```python
from build123d import *

# Parameters (mm, degrees)
MODEL_R             = 42.5
MODEL_R_2           = 5.5
MODEL_R_3           = 2.75
MODEL_R_4           = 3.1
MODEL_W             = 25.4
MODEL_H             = 25.4
BOSS_EXTRUDE1_DEPTH = 6.6


with BuildPart() as part:
    # Model → Boss-Extrude1 (new body)
    with BuildSketch(Plane.XY):
        with BuildLine():
            Line((187.8, 2), (187.8, 24.665))
            Line((187.8, 24.665), (176.8, 24.665))
            Line((176.8, 24.665), (176.8, 23.08))
            ThreePointArc((176.8, 23.08), (176.653553391, 22.726446609), (176.3, 22.58))
            Line((176.3, 22.58), (172.3, 22.58))
            ThreePointArc((172.3, 22.58), (171.946446609, 22.726446609), (171.8, 23.08))
            Line((171.8, 23.08), (171.8, 24.665))
            Line((171.8, 24.665), (167.3, 24.665))
            ThreePointArc((167.3, 24.665), (166.946446609, 24.811446609), (166.8, 25.165))
            Line((166.8, 25.165), (166.8, 27.715))
            ThreePointArc((166.8, 27.715), (166.946446609, 28.068553391), (167.3, 28.215))
            Line((167.3, 28.215), (171.8, 28.215))
            Line((171.8, 28.215), (171.8, 29.8))
            ThreePointArc((171.8, 29.8), (171.946446609, 30.153553391), (172.3, 30.3))
            Line((172.3, 30.3), (176.3, 30.3))
            ThreePointArc((176.3, 30.3), (176.653553391, 30.153553391), (176.8, 29.8))
            Line((176.8, 29.8), (176.8, 28.215))
            Line((176.8, 28.215), (187.8, 28.215))
            Line((187.8, 28.215), (187.8, 42.8))
            Line((187.8, 42.8), (191.8, 42.8))
            ThreePointArc((191.8, 42.8), (193.567766953, 43.532233047), (194.3, 45.3))
            Line((194.3, 45.3), (194.3, 55.3))
            ThreePointArc((194.3, 55.3), (193.567766953, 57.067766953), (191.8, 57.8))
            Line((191.8, 57.8), (187.8, 57.8))
            Line((187.8, 57.8), (187.8, 118.92))
            Line((187.8, 118.92), (191.8, 118.92))
            ThreePointArc((191.8, 118.92), (193.567766953, 119.652233047), (194.3, 121.42))
            Line((194.3, 121.42), (194.3, 131.42))
            ThreePointArc((194.3, 131.42), (193.567766953, 133.187766953), (191.8, 133.92))
            Line((191.8, 133.92), (187.8, 133.92))
            Line((187.8, 133.92), (187.8, 152.92))
            Line((187.8, 152.92), (176.8, 152.92))
            Line((176.8, 152.92), (176.8, 151.335))
            ThreePointArc((176.8, 151.335), (176.653553391, 150.981446609), (176.3, 150.835))
            Line((176.3, 150.835), (172.3, 150.835))
            ThreePointArc((172.3, 150.835), (171.946446609, 150.981446609), (171.8, 151.335))
            Line((171.8, 151.335), (171.8, 152.92))
            Line((171.8, 152.92), (167.3, 152.92))
            ThreePointArc((167.3, 152.92), (166.946446609, 153.066446609), (166.8, 153.42))
            Line((166.8, 153.42), (166.8, 155.97))
            ThreePointArc((166.8, 155.97), (166.946446609, 156.323553391), (167.3, 156.47))
            Line((167.3, 156.47), (171.8, 156.47))
            Line((171.8, 156.47), (171.8, 158.055))
            ThreePointArc((171.8, 158.055), (171.946446609, 158.408553391), (172.3, 158.555))
            Line((172.3, 158.555), (176.3, 158.555))
            ThreePointArc((176.3, 158.555), (176.653553391, 158.408553391), (176.8, 158.055))
            Line((176.8, 158.055), (176.8, 156.47))
            Line((176.8, 156.47), (187.8, 156.47))
            Line((187.8, 156.47), (187.8, 169.42))
            Line((187.8, 169.42), (185.8, 171.42))
            Line((185.8, 171.42), (113.770001664, 171.42))
            Line((113.770001664, 171.42), (113.770001664, 158.72))
            Line((113.770001664, 158.72), (106.910001664, 158.72))
            Line((106.910001664, 158.72), (106.910001664, 171.42))
            Line((106.910001664, 171.42), (81.510001665, 171.42))
            Line((81.510001665, 171.42), (81.510001665, 158.72))
            Line((81.510001665, 158.72), (74.650001665, 158.72))
            Line((74.650001665, 158.72), (74.650001665, 171.42))
            Line((74.650001665, 171.42), (2, 171.42))
            Line((2, 171.42), (0, 169.42))
            Line((0, 169.42), (0, 156.47))
            Line((0, 156.47), (11, 156.47))
            Line((11, 156.47), (11, 158.055))
            ThreePointArc((11, 158.055), (11.146446609, 158.408553391), (11.5, 158.555))
            Line((11.5, 158.555), (15.5, 158.555))
            ThreePointArc((15.5, 158.555), (15.853553391, 158.408553391), (16, 158.055))
            Line((16, 158.055), (16, 156.47))
            Line((16, 156.47), (20.5, 156.47))
            ThreePointArc((20.5, 156.47), (20.853553391, 156.323553391), (21, 155.97))
            Line((21, 155.97), (21, 153.42))
            ThreePointArc((21, 153.42), (20.853553391, 153.066446609), (20.5, 152.92))
            Line((20.5, 152.92), (16, 152.92))
            Line((16, 152.92), (16, 151.335))
            ThreePointArc((16, 151.335), (15.853553391, 150.981446609), (15.5, 150.835))
            Line((15.5, 150.835), (11.5, 150.835))
            ThreePointArc((11.5, 150.835), (11.146446609, 150.981446609), (11, 151.335))
            Line((11, 151.335), (11, 152.92))
            Line((11, 152.92), (0, 152.92))
            Line((0, 152.92), (0, 133.92))
            Line((0, 133.92), (-4, 133.92))
            ThreePointArc((-4, 133.92), (-5.767766953, 133.187766953), (-6.5, 131.42))
            Line((-6.5, 131.42), (-6.5, 121.42))
            ThreePointArc((-6.5, 121.42), (-5.767766953, 119.652233047), (-4, 118.92))
            Line((-4, 118.92), (0, 118.92))
            Line((0, 118.92), (0, 57.8))
            Line((0, 57.8), (-4, 57.8))
            ThreePointArc((-4, 57.8), (-5.767766953, 57.067766953), (-6.5, 55.3))
            Line((-6.5, 55.3), (-6.5, 45.3))
            ThreePointArc((-6.5, 45.3), (-5.767766953, 43.532233047), (-4, 42.8))
            Line((-4, 42.8), (0, 42.8))
            Line((0, 42.8), (0, 28.215))
            Line((0, 28.215), (11, 28.215))
            Line((11, 28.215), (11, 29.8))
            ThreePointArc((11, 29.8), (11.146446609, 30.153553391), (11.5, 30.3))
            Line((11.5, 30.3), (15.5, 30.3))
            ThreePointArc((15.5, 30.3), (15.853553391, 30.153553391), (16, 29.8))
            Line((16, 29.8), (16, 28.215))
            Line((16, 28.215), (20.5, 28.215))
            ThreePointArc((20.5, 28.215), (20.853553391, 28.068553391), (21, 27.715))
            Line((21, 27.715), (21, 25.165))
            ThreePointArc((21, 25.165), (20.853553391, 24.811446609), (20.5, 24.665))
            Line((20.5, 24.665), (16, 24.665))
            Line((16, 24.665), (16, 23.08))
            ThreePointArc((16, 23.08), (15.853553391, 22.726446609), (15.5, 22.58))
            Line((15.5, 22.58), (11.5, 22.58))
            ThreePointArc((11.5, 22.58), (11.146446609, 22.726446609), (11, 23.08))
            Line((11, 23.08), (11, 24.665))
            Line((11, 24.665), (0, 24.665))
            Line((0, 24.665), (0, 2))
            Line((0, 2), (2, 0))
            Line((2, 0), (25.4, 0))
            Line((25.4, 0), (25.4, -4))
            ThreePointArc((25.4, -4), (26.132233047, -5.767766953), (27.9, -6.5))
            Line((27.9, -6.5), (37.9, -6.5))
            ThreePointArc((37.9, -6.5), (39.667766953, -5.767766953), (40.4, -4))
            Line((40.4, -4), (40.4, 0))
            Line((40.4, 0), (147.4, 0))
            Line((147.4, 0), (147.4, -4))
            ThreePointArc((147.4, -4), (148.132233047, -5.767766953), (149.9, -6.5))
            Line((149.9, -6.5), (159.9, -6.5))
            ThreePointArc((159.9, -6.5), (161.667766953, -5.767766953), (162.4, -4))
            Line((162.4, -4), (162.4, 0))
            Line((162.4, 0), (185.8, 0))
            Line((185.8, 0), (187.8, 2))
        make_face()
        with Locations((94.21, 58.872106781)):
            Circle(MODEL_R, mode=Mode.SUBTRACT)
        with Locations((139.852001664, 123.924806781)):
            Circle(MODEL_R_2, mode=Mode.SUBTRACT)
        with Locations((48.39651697, 124.09019794)):
            Circle(MODEL_R_2, mode=Mode.SUBTRACT)
        with Locations((182.8, 123.5)):
            Circle(MODEL_R_3, mode=Mode.SUBTRACT)
        with Locations((5.447263086, 123.820730625)):
            Circle(MODEL_R_3, mode=Mode.SUBTRACT)
        with Locations((162.4, 58.872106781)):
            Circle(MODEL_R_4, mode=Mode.SUBTRACT)
        with Locations((25.4, 58.872106781)):
            Circle(MODEL_R_4, mode=Mode.SUBTRACT)
        with Locations((94.210001664, 123.924806781)):
            Rectangle(MODEL_W, MODEL_H, mode=Mode.SUBTRACT)
        with BuildLine():
            Line((183.8, 82.4), (183.8, 80))
            ThreePointArc((183.8, 80), (184.55, 79.25), (185.3, 80))
            Line((185.3, 80), (185.3, 82.4))
            ThreePointArc((185.3, 82.4), (184.55, 83.15), (183.8, 82.4))
        make_face(mode=Mode.SUBTRACT)
        with BuildLine():
            Line((176.8, 82.4), (176.8, 80))
            ThreePointArc((176.8, 80), (177.55, 79.25), (178.3, 80))
            Line((178.3, 80), (178.3, 82.4))
            ThreePointArc((178.3, 82.4), (177.55, 83.15), (176.8, 82.4))
        make_face(mode=Mode.SUBTRACT)
        with BuildLine():
            Line((9.798580907, 82.704723605), (9.789900455, 80.304739303))
            ThreePointArc((9.789900455, 80.304739303), (10.537182908, 79.552031568), (11.289890644, 80.299314021))
            Line((11.289890644, 80.299314021), (11.298571096, 82.699298323))
            ThreePointArc((11.298571096, 82.699298323), (10.551288643, 83.452006058), (9.798580907, 82.704723605))
        make_face(mode=Mode.SUBTRACT)
        with BuildLine():
            Line((2.798626693, 82.730041591), (2.789946241, 80.330057289))
            ThreePointArc((2.789946241, 80.330057289), (3.537228694, 79.577349553), (4.28993643, 80.324632006))
            Line((4.28993643, 80.324632006), (4.298616882, 82.724616308))
            ThreePointArc((4.298616882, 82.724616308), (3.551334429, 83.477324044), (2.798626693, 82.730041591))
        make_face(mode=Mode.SUBTRACT)
    extrude(amount=BOSS_EXTRUDE1_DEPTH)


solid = part.part
```
Model file for the job. Use its own axes, mm. A direction names the side the tool comes from. Give positions to 0.01 mm unless a question says otherwise; leave off trailing zeros. Write each loop counter-clockwise with the first axis right and the second up, starting at its lowest first coordinate (ties: lowest second). Pieces come first, ordered by that corner, then holes. Notation, with made-up numbers: (81, 45) -> (133, 45) arc R21 ccw to (133, 71) -> close; hole circle Ø10 at (-39, 69.5). An arc over 180 degrees is marked (long way). Use CSV: the item, a comma, the result in double quotes. Start each with the question number.
1) Cut at B-B on x = 94.5. List the corners of the cut face in (y, z), plus the area to 3 significant figures.
2) Two-plate mould, pull along X, no slides. Class faces 6 (the flat face through (0, 89, 3)), 7 (the flat face through (113.77, 165, 3)), 8 (the flat face through (5, 156.47, 3)): released by +X, released by -X, zero draft, split by the parting line, or undercut.
3) Cut at A-A on x = 63. List the corners of the cut face in (y, z), plus the area to 3 significant figures.
4) Tool access for faces 1 (the flat face through (0, 36, 3)), 2 (the flat face through (106.91, 124, 3)), 3 (the flat face through (78, 158.72, 3)), 4 (the flat face through (182, 28.215, 3)), 5 (the flat face through (6, 24.665, 3)): list every direction of +Z, -Z, +X, -X, +Y, -Y with a clear straight run to the whole face (end or side of a thin tool).
5) Drill centre lines: L1, parallel to Y at x = 182.8, z = 3 (3 decimals); L2, parallel to Y at x = 12.5, z = 3.25 (3 decimals); L3, parallel to X at y = 57, z = 3.5. Where is each one in solid material? Low to high.
6) Pin check, flat tips, straight feed: P1, Ø0.7, axis at y = 81.5, z = 3.5, coming from the +X side; P2, Ø1, axis at x = 54, z = 3, coming from the -Y side; P3, Ø1.3, axis at y = 24, z = 4, coming from the -X side. Stop position of each tip, or through.
7) Cut at C-C on z = 4. Count the separate pieces of the cut face and the enclosed holes in it, plus the area to 3 significant figures.
Final values:
1,outline,"(0, 0) -> (16.37, 0) -> (16.37, 6.6) -> (0, 6.6) -> close; (101.37, 0) -> (111.22, 0) -> (111.22, 6.6) -> (101.37, 6.6) -> close; (136.62, 0) -> (171.42, 0) -> (171.42, 6.6) -> (136.62, 6.6) -> close"
1,area,"403 mm2"
2,face 6,"released by -X"
2,face 7,"undercut"
2,face 8,"zero draft"
3,outline,"(0, 0) -> (30.02, 0) -> (30.02, 6.6) -> (0, 6.6) -> close; (87.72, 0) -> (171.42, 0) -> (171.42, 6.6) -> (87.72, 6.6) -> close"
3,area,"751 mm2"
4,face 1,"+Z, -Z, -X, -Y"
4,face 2,"+Z, -Z"
4,face 3,"+Z, -Z, +Y"
4,face 4,"+Z, -Z, +X"
4,face 5,"+Z, -Z, -X"
5,L1,"y = 0 to 24.665, 28.215 to 120.75, 126.25 to 152.92, 156.47 to 171.42"
5,L2,"y = 0 to 22.58, 30.3 to 150.835, 158.555 to 171.42"
5,L3,"x = -5.83 to 22.93, 27.87 to 51.75, 136.67 to 159.93, 164.87 to 193.63"
6,P1,"stops at x = 187.8"
6,P2,"stops at y = 0"
6,P3,"stops at x = 0"
7,separate pieces,"1"
7,enclosed holes,"12"
7,area,"25,600 mm2"
